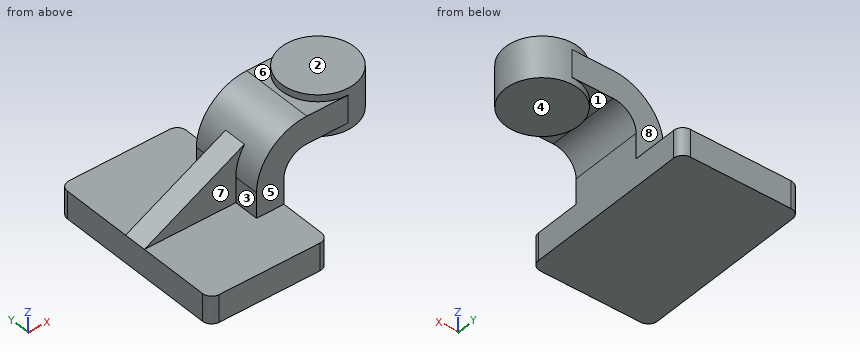
```python
from build123d import *

# Parameters (mm, degrees)
F1_DEPTH = 63.5
F2_DEPTH = 25.4
F3_DEPTH = 7.9375
F5_R     = 6.35


with BuildPart() as f1:
    # F0 (on Front) → F1 (new body, symmetric)
    with BuildSketch(Plane.XZ):
        Polygon((22.225, 9.525), (-41.275, 9.525), (-41.275, -9.525), (41.275, -9.525), (41.275, 9.525), align=None)
    extrude(amount=F1_DEPTH, both=True)

    # F0 (on Front) → F2 (join, symmetric)
    with BuildSketch(Plane.XZ):
        Polygon((85.725, 61.9252), (60.325, 61.9252), (60.325, 42.8752), (80.5717907127, 42.8752), (85.725, 42.8752), align=None)
        with BuildLine():
            Line((22.225, 27.0002), (22.225, 9.525))
            Line((22.225, 9.525), (41.275, 9.525))
            Line((41.275, 9.525), (41.275, 27.0002))
            ThreePointArc((41.275, 27.0002), (45.9246798487, 38.2255201513), (57.15, 42.8752))
            Line((57.15, 42.8752), (60.325, 42.8752))
            Line((60.325, 42.8752), (60.325, 61.9252))
            Line((60.325, 61.9252), (57.15, 61.9252))
            add(Edge.make_bspline(
                [(28.1752493255, 46.4994166087), (37.8334995503, 51.6413444058), (47.4917497752, 56.7832722029), (57.15, 61.9252)],
                knots=[78.6793785876, 78.6793785876, 78.6793785876, 78.6793785876, 111.5045361635, 111.5045361635, 111.5045361635, 111.5045361635], degree=3))
            ThreePointArc((28.1752493255, 46.4994166087), (23.7456680032, 37.1936404813), (22.225, 27.0002))
        make_face()
        with BuildLine():
            ThreePointArc((57.15, 61.9252), (40.737421212, 57.8284805639), (28.1752493255, 46.4994166087))
            add(Edge.make_bspline(
                [(28.1752493255, 46.4994166087), (37.8334995503, 51.6413444058), (47.4917497752, 56.7832722029), (57.15, 61.9252)],
                knots=[78.6793785876, 78.6793785876, 78.6793785876, 78.6793785876, 111.5045361635, 111.5045361635, 111.5045361635, 111.5045361635], degree=3))
        make_face()
    extrude(amount=F2_DEPTH, both=True)

    # F0 (on Front) → F3 (join, symmetric)
    with BuildSketch(Plane.XZ):
        with BuildLine():
            add(Edge.make_bspline(
                [(-41.275, 9.525), (-18.1249168915, 21.8498055362), (5.025166217, 34.1746110724), (28.1752493255, 46.4994166087)],
                knots=[0, 0, 0, 0, 78.6793785876, 78.6793785876, 78.6793785876, 78.6793785876], degree=3))
            Line((-41.275, 9.525), (22.225, 9.525))
            Line((22.225, 9.525), (22.225, 27.0002))
            ThreePointArc((22.225, 27.0002), (23.7456680032, 37.1936404813), (28.1752493255, 46.4994166087))
        make_face()
    extrude(amount=F3_DEPTH, both=True)

    # F0 (on Front) → F4 (revolve)
    with BuildSketch(Plane.XZ):
        Polygon((85.725, 66.675), (85.725, 61.9252), (85.725, 42.8752), (85.725, 38.1), (111.125, 38.1), (111.125, 66.675), align=None)
    revolve(axis=Axis((85.725, 0, 52.3875), (0, 0, -1)))

    # F5
    f5_edges = [f1.edges().sort_by_distance(p)[0] for p in [
        (-41.275, -63.5, 0),
        (41.275, -63.5, 0),
        (41.275, 63.5, 0),
        (-41.275, 63.5, 0),
    ]]
    fillet(f5_edges, radius=F5_R)


solid = f1.part
```
Geometry check sheet. Reference: the model listing, model coordinates, mm. Face numbers are marked on the shaded views. A direction names the side the tool comes from. Coordinates: 2 decimals unless noted, no trailing zeros. Write each loop counter-clockwise with the first axis right and the second up, starting at its lowest first coordinate (ties: lowest second). Pieces come first, ordered by that corner, then holes. Notation, with made-up numbers: M 66,-30 L 70,-30 A26 cw 70,-6 Z; hole C 68.5,1 d6. An arc over 180 degrees is marked long. Answer as a JSON object with one key per item and string values.
1. Section check D-D, the plane y = 52.5. Enter the section's corners in (x, z) (3 decimals), plus the area to 3 significant figures.
Answers below:
{"outline": "M -41.275,-9.525 L 41.275,-9.525 L 41.275,9.525 L -41.275,9.525 Z", "area": "1,570 mm²"}
2. Go/stop test with flat-tipped pins: pin 1 Ø4 at (y, z) = (50, 1) entering from +X (3 decimals); pin 2 Ø8.5 at (y, z) = (21, 19.5) entering from -X (3 decimals); pin 3 Ø10 at (y, z) = (-14, 45) entering from +X. Record where each tip stops, or that it passes through.
Answers below:
{"pin 1": "stops at x = 41.275", "pin 2": "stops at x = 22.225", "pin 3": "stops at x = 109.48"}
3. Section check A-A, the plane y = 0. Enter the section's corners in (x, z) (3 decimals).
Answers below:
{"outline": "M -41.275,-9.525 L 41.275,-9.525 L 41.275,27 A15.875 cw 57.15,42.875 L 60.325,42.875 L 60.325,38.1 L 111.125,38.1 L 111.125,66.675 L 60.325,66.675 L 60.325,61.925 L 57.15,61.925 A34.925 ccw 28.175,46.499 L -41.275,9.525 Z"}
4. Section check B-B, the plane z = 5.5. Enter the section's corners in (x, y) (3 decimals), plus the area to 3 significant figures.
Answers below:
{"outline": "M -41.275,-57.15 A6.35 ccw -34.925,-63.5 L 34.925,-63.5 A6.35 ccw 41.275,-57.15 L 41.275,57.15 A6.35 ccw 34.925,63.5 L -34.925,63.5 A6.35 ccw -41.275,57.15 Z", "area": "10,400 mm²"}
5. Tool access check on the marked faces 4, 5, 6, 7 and 8. Record the directions out of +Z, -Z, +X, -X, +Y, -Y that give a thin tool (end or side, any length) a straight path to the whole face; none if there is none.
Answers below:
{"face 4": "-Z, +X, +Y, -Y", "face 5": "+Z, +X, -X, -Y", "face 6": "+Z, -X", "face 7": "+Z, -X, -Y", "face 8": "+Z, +X, -X, +Y"}
6. Draft check along X on the marked faces 1, 2 and 3. Enter one of: released by +X, released by -X, zero draft, split by the parting line, or undercut.
Answers below:
{"face 1": "undercut", "face 2": "zero draft", "face 3": "released by -X"}
7. Section check C-C, the plane x = 74. Enter the section's corners in (y, z) (3 decimals).
Answers below:
{"outline": "M -25.4,42.875 L -22.532,42.875 L -22.532,38.1 L 22.532,38.1 L 22.532,42.875 L 25.4,42.875 L 25.4,61.925 L 22.532,61.925 L 22.532,66.675 L -22.532,66.675 L -22.532,61.925 L -25.4,61.925 Z"}
8. Scan lines: L1, parallel to Z at x = 4, y = 10 (3 decimals); L2, parallel to Z at x = 71, y = 23; L3, parallel to X at y = 45.5, z = 6 (3 decimals). Record each from-to range of solid material in increasing order.
Answers below:
{"L1": "z = -9.525 to 9.525", "L2": "z = 42.88 to 61.93", "L3": "x = -41.275 to 41.275"}
